Geometry check sheet. Reference: the model listing, model coordinates, mm. Face numbers are marked on the shaded views. A direction names the side the tool comes from. Round coordinates to 2 decimals unless told otherwise and drop trailing zeros. Loops run counter-clockwise (first coordinate to the right, second up) from the corner with the lowest first, then second, coordinate; pieces in that order, holes last.
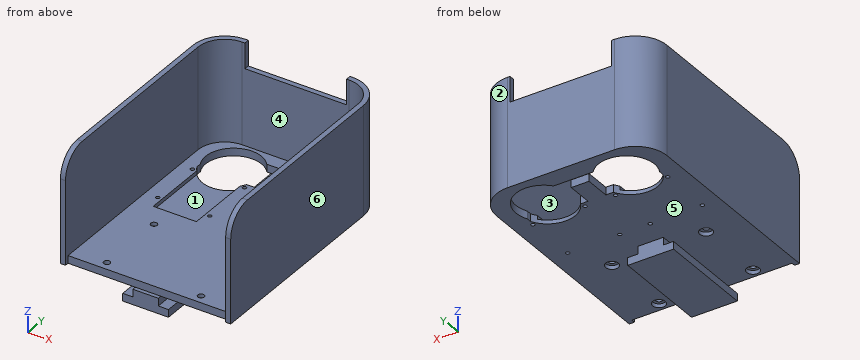
```python
from build123d import *

# Parameters (mm, degrees)
SKETCH_1_W           = 63
SKETCH_1_H           = 70
EXTRUDE_1_DEPTH      = 3
CUT_EXTRUDE_1_REACH  = 96.223
SKETCH_2_R           = 0.75
SKETCH_3_W           = 17
SKETCH_3_H           = 1.5
CUT_EXTRUDE_2_DEPTH  = 28
SKETCH_4_R           = 11
CUT_EXTRUDE_3_DEPTH  = 95.223139409
CUT_EXTRUDE_5_REACH  = 96.223
SKETCH_6_R           = 1.25
SKETCH_7_R           = 2.5
CUT_EXTRUDE_6_DEPTH  = 1.5
SKETCH_9_W           = 7
SKETCH_9_H           = 10
EXTRUDE_2_DEPTH      = 3
SKETCH_10_W          = 10
SKETCH_10_H          = 38
EXTRUDE_3_DEPTH      = 3
SKETCH_11_W          = 18
SKETCH_11_H          = 38
EXTRUDE_4_DEPTH      = 3
SKETCH_12_W          = 2
SKETCH_12_H          = 70
EXTRUDE_5_DEPTH      = 43
SWEEP_1_DEPTH        = 43
SWEEP_1_2_DEPTH      = 3
CUT_EXTRUDE_7_DEPTH  = 122.249642508
SKETCH_16_R          = 11
CUT_EXTRUDE_9_DEPTH  = 120.11538863
SKETCH_21_W          = 63
SKETCH_21_H          = 1.5
CUT_EXTRUDE_10_DEPTH = 3
CUT_EXTRUDE_11_REACH = 122.156
SKETCH_23_W          = 40
SKETCH_23_H          = 10


# Read off the part's stored shape, not the designer's step: the sweep step
with BuildPart() as part:
    # Sketch 1 → Extrude 1 (new body)
    with BuildSketch(Plane.XY):
        with Locations((31.5, 35)):
            Rectangle(SKETCH_1_W, SKETCH_1_H)
    extrude(amount=EXTRUDE_1_DEPTH)

    # Sketch 2 → Cut-Extrude 1 (cut, up to next)
    with BuildSketch(Plane.XY.offset(3), mode=Mode.PRIVATE) as cut_extrude_1_sk1:
        with Locations((5, 68)):
            Circle(SKETCH_2_R)
    cut_extrude_1_tool1 = extrude(cut_extrude_1_sk1.sketch, amount=-CUT_EXTRUDE_1_REACH, mode=Mode.PRIVATE) & part.part
    # Sketch 2 → Cut-Extrude 1 (cut, up to next)
    with BuildSketch(Plane.XY.offset(3), mode=Mode.PRIVATE) as cut_extrude_1_sk2:
        with Locations((5, 47.3)):
            Circle(SKETCH_2_R)
    cut_extrude_1_tool2 = extrude(cut_extrude_1_sk2.sketch, amount=-CUT_EXTRUDE_1_REACH, mode=Mode.PRIVATE) & part.part
    # Sketch 2 → Cut-Extrude 1 (cut, up to next)
    with BuildSketch(Plane.XY.offset(3), mode=Mode.PRIVATE) as cut_extrude_1_sk3:
        with Locations((25.5, 47.3)):
            Circle(SKETCH_2_R)
    cut_extrude_1_tool3 = extrude(cut_extrude_1_sk3.sketch, amount=-CUT_EXTRUDE_1_REACH, mode=Mode.PRIVATE) & part.part
    # Sketch 2 → Cut-Extrude 1 (cut, up to next)
    with BuildSketch(Plane.XY.offset(3), mode=Mode.PRIVATE) as cut_extrude_1_sk4:
        with Locations((25.5, 68)):
            Circle(SKETCH_2_R)
    cut_extrude_1_tool4 = extrude(cut_extrude_1_sk4.sketch, amount=-CUT_EXTRUDE_1_REACH, mode=Mode.PRIVATE) & part.part
    cut_extrude_1_1 = cut_extrude_1_tool1.solids().sort_by_distance((5, 68, 3))[0]
    add(cut_extrude_1_1, mode=Mode.SUBTRACT)
    cut_extrude_1_2 = cut_extrude_1_tool2.solids().sort_by_distance((5, 47.3, 3))[0]
    add(cut_extrude_1_2, mode=Mode.SUBTRACT)
    cut_extrude_1_3 = cut_extrude_1_tool3.solids().sort_by_distance((25.5, 47.3, 3))[0]
    add(cut_extrude_1_3, mode=Mode.SUBTRACT)
    cut_extrude_1_4 = cut_extrude_1_tool4.solids().sort_by_distance((25.5, 68, 3))[0]
    add(cut_extrude_1_4, mode=Mode.SUBTRACT)
    cut_extrude_1 = cut_extrude_1_1 + cut_extrude_1_2 + cut_extrude_1_3 + cut_extrude_1_4  # Cut-Extrude 1 as one shape, for the pattern or mirror that repeats it

    # Sketch 3 → Cut-Extrude 2 (cut)
    with BuildSketch(Plane(origin=(0, 70, 0), x_dir=(1, 0, 0), z_dir=(0, 1, 0))):
        with Locations((15.25, -2.25)):
            Rectangle(SKETCH_3_W, SKETCH_3_H)
    cut_extrude_2 = extrude(amount=-CUT_EXTRUDE_2_DEPTH, mode=Mode.SUBTRACT)

    # Sketch 4 → Cut-Extrude 3 (cut, through all)
    with BuildSketch(Plane(origin=(0, 0, 0), x_dir=(-1, 0, 0), z_dir=(0, 0, -1))):
        with Locations((-15.25, 75)):
            Circle(SKETCH_4_R)
    cut_extrude_3 = extrude(amount=-CUT_EXTRUDE_3_DEPTH, mode=Mode.SUBTRACT)

    # Mirror 1: Cut-Extrude 1, Cut-Extrude 2, Cut-Extrude 3 across plane
    add(cut_extrude_1.mirror(Plane.ZY.offset(-31.5)), mode=Mode.SUBTRACT)
    add(cut_extrude_2.mirror(Plane.ZY.offset(-31.5)), mode=Mode.SUBTRACT)
    add(cut_extrude_3.mirror(Plane.ZY.offset(-31.5)), mode=Mode.SUBTRACT)

    # Sketch 6 → Cut-Extrude 5 (cut, up to next)
    with BuildSketch(Plane(origin=(0, 0, 0), x_dir=(-1, 0, 0), z_dir=(0, 0, -1)), mode=Mode.PRIVATE) as cut_extrude_5_sk1:
        with Locations((-50, 5)):
            Circle(SKETCH_6_R)
    cut_extrude_5_tool1 = extrude(cut_extrude_5_sk1.sketch, amount=-CUT_EXTRUDE_5_REACH, mode=Mode.PRIVATE) & part.part
    # Sketch 6 → Cut-Extrude 5 (cut, up to next)
    with BuildSketch(Plane(origin=(0, 0, 0), x_dir=(-1, 0, 0), z_dir=(0, 0, -1)), mode=Mode.PRIVATE) as cut_extrude_5_sk2:
        with Locations((-50, 33)):
            Circle(SKETCH_6_R)
    cut_extrude_5_tool2 = extrude(cut_extrude_5_sk2.sketch, amount=-CUT_EXTRUDE_5_REACH, mode=Mode.PRIVATE) & part.part
    # Sketch 6 → Cut-Extrude 5 (cut, up to next)
    with BuildSketch(Plane(origin=(0, 0, 0), x_dir=(-1, 0, 0), z_dir=(0, 0, -1)), mode=Mode.PRIVATE) as cut_extrude_5_sk3:
        with Locations((-13, 33)):
            Circle(SKETCH_6_R)
    cut_extrude_5_tool3 = extrude(cut_extrude_5_sk3.sketch, amount=-CUT_EXTRUDE_5_REACH, mode=Mode.PRIVATE) & part.part
    # Sketch 6 → Cut-Extrude 5 (cut, up to next)
    with BuildSketch(Plane(origin=(0, 0, 0), x_dir=(-1, 0, 0), z_dir=(0, 0, -1)), mode=Mode.PRIVATE) as cut_extrude_5_sk4:
        with Locations((-13, 5)):
            Circle(SKETCH_6_R)
    cut_extrude_5_tool4 = extrude(cut_extrude_5_sk4.sketch, amount=-CUT_EXTRUDE_5_REACH, mode=Mode.PRIVATE) & part.part
    add(cut_extrude_5_tool1.solids().sort_by_distance((50, 5, 0))[0], mode=Mode.SUBTRACT)
    add(cut_extrude_5_tool2.solids().sort_by_distance((50, 33, 0))[0], mode=Mode.SUBTRACT)
    add(cut_extrude_5_tool3.solids().sort_by_distance((13, 33, 0))[0], mode=Mode.SUBTRACT)
    add(cut_extrude_5_tool4.solids().sort_by_distance((13, 5, 0))[0], mode=Mode.SUBTRACT)

    # Sketch 7 → Cut-Extrude 6 (cut)
    with BuildSketch(Plane(origin=(0, 0, 0), x_dir=(-1, 0, 0), z_dir=(0, 0, -1))):
        with Locations((-50, 33)):
            Circle(SKETCH_7_R)
        with Locations((-13, 33)):
            Circle(SKETCH_7_R)
        with Locations((-13, 5)):
            Circle(SKETCH_7_R)
        with Locations((-50, 5)):
            Circle(SKETCH_7_R)
    extrude(amount=-CUT_EXTRUDE_6_DEPTH, mode=Mode.SUBTRACT)

    # Sketch 9 → Extrude 2 (add)
    with BuildSketch(Plane(origin=(0, 0, 0), x_dir=(-1, 0, 0), z_dir=(0, 0, -1))):
        with Locations((-31.5, 75)):
            Rectangle(SKETCH_9_W, SKETCH_9_H)
    extrude(amount=-EXTRUDE_2_DEPTH)

    # Sketch 10 → Extrude 3 (add)
    with BuildSketch(Plane(origin=(0, 0, 0), x_dir=(-1, 0, 0), z_dir=(0, 0, -1))):
        with Locations((-31.5, 19)):
            Rectangle(SKETCH_10_W, SKETCH_10_H)
    extrude(amount=EXTRUDE_3_DEPTH)

    # Sketch 11 → Extrude 4 (add)
    with BuildSketch(Plane(origin=(0, 0, -3), x_dir=(-1, 0, 0), z_dir=(0, 0, -1))):
        with Locations((-31.5, 19)):
            Rectangle(SKETCH_11_W, SKETCH_11_H)
    extrude(amount=EXTRUDE_4_DEPTH)

    # Sketch 12 → Extrude 5 (add)
    with BuildSketch(Plane(origin=(0, 0, 0), x_dir=(-1, 0, 0), z_dir=(0, 0, -1))):
        with Locations((-64, 35)):
            Rectangle(SKETCH_12_W, SKETCH_12_H)
        with Locations((1, 35)):
            Rectangle(SKETCH_12_W, SKETCH_12_H)
    extrude(amount=-EXTRUDE_5_DEPTH)

    # Sweep 1 outline → Sweep 1 (add)
    with BuildSketch(Plane.XY):
        with BuildLine():
            ThreePointArc((52.547958971, 89.452041029), (59.93866806, 86.390709089), (63, 79))
            Line((63, 79), (63, 70))
            Line((63, 70), (65, 70))
            Line((65, 70), (65, 79))
            ThreePointArc((65, 79), (61.352881622, 87.804922651), (52.547958971, 91.452041029))
            Line((52.547958971, 91.452041029), (10.452041029, 91.452041029))
            ThreePointArc((10.452041029, 91.452041029), (1.647118378, 87.804922651), (-2, 79))
            Line((-2, 79), (-2, 70))
            Line((-2, 70), (0, 70))
            Line((0, 70), (0, 79))
            ThreePointArc((0, 79), (3.06133194, 86.390709089), (10.452041029, 89.452041029))
            Line((10.452041029, 89.452041029), (52.547958971, 89.452041029))
        make_face()
    extrude(amount=SWEEP_1_DEPTH)

    # Sweep 1 2 outline → Sweep 1 2 (add)
    with BuildSketch(Plane.XY):
        with BuildLine():
            Line((63, 70), (63, 79))
            ThreePointArc((63, 79), (59.93866806, 86.390709089), (52.547958971, 89.452041029))
            Line((52.547958971, 89.452041029), (10.452041029, 89.452041029))
            ThreePointArc((10.452041029, 89.452041029), (3.06133194, 86.390709089), (0, 79))
            Line((0, 79), (0, 70))
            Line((0, 70), (5.452041029, 70))
            Line((5.452041029, 70), (5.452041029, 79))
            ThreePointArc((5.452041029, 79), (6.916507123, 82.535533906), (10.452041029, 84))
            Line((10.452041029, 84), (52.547958971, 84))
            ThreePointArc((52.547958971, 84), (56.083492877, 82.535533906), (57.547958971, 79))
            Line((57.547958971, 79), (57.547958971, 70))
            Line((57.547958971, 70), (63, 70))
        make_face()
    extrude(amount=SWEEP_1_2_DEPTH)

    # Sketch 15 → Cut-Extrude 7 (cut, through all)
    with BuildSketch(Plane.ZY.offset(2)):
        with BuildLine():
            ThreePointArc((43, 10), (40.071067812, 2.928932188), (33, 0))
            Line((33, 0), (43, 0))
            Line((43, 0), (43, 10))
        make_face()
    extrude(amount=-CUT_EXTRUDE_7_DEPTH, mode=Mode.SUBTRACT)

    # Sketch 16 → Cut-Extrude 9 (cut, through all)
    with BuildSketch(Plane.XY.offset(3)):
        with Locations((15.25, 77)):
            Circle(SKETCH_16_R)
        with Locations((47.75, 77)):
            Circle(SKETCH_16_R)
    extrude(amount=-CUT_EXTRUDE_9_DEPTH, mode=Mode.SUBTRACT)

    # Sketch 21 → Cut-Extrude 10 (cut)
    with BuildSketch(Plane.XY.offset(3)):
        with Locations((31.5, 0.75)):
            Rectangle(SKETCH_21_W, SKETCH_21_H)
    extrude(amount=-CUT_EXTRUDE_10_DEPTH, mode=Mode.SUBTRACT)

    # Sketch 23 → Cut-Extrude 11 (cut, up to next)
    with BuildSketch(Plane(origin=(0, 91.452041029, 0), x_dir=(1, 0, 0), z_dir=(0, 1, 0)), mode=Mode.PRIVATE) as cut_extrude_11_sk1:
        with Locations((31.5, -38)):
            Rectangle(SKETCH_23_W, SKETCH_23_H)
    cut_extrude_11_tool1 = extrude(cut_extrude_11_sk1.sketch, amount=-CUT_EXTRUDE_11_REACH, mode=Mode.PRIVATE) & part.part
    add(cut_extrude_11_tool1.solids().sort_by_distance((31.5, 91.452041, 38))[0], mode=Mode.SUBTRACT)


solid = part.part
```
1) Mould release check, pull along X, two halves, no side actions. Record for the marked faces 4, 5 and 6: +X half, -X half, draft (parallel to the pull), parting line (faces both ways), or undercut.
Report:
face 4: undercut
face 5: draft
face 6: +X half
2) Sectioned sample at A-A, the plane y = 33. State how many separate pieces and enclosed holes the cut face has, then the cut area to 4 significant figures.
Report:
separate pieces: 3
enclosed holes: 0
area: 422.5 mm2
3) Scan lines: line 1 along X through (y, z) = (19, 12); line 2 along Y through (x, z) = (37, 2); line 3 along Y through (x, z) = (37.5, 1.65). Record each from-to range of solid material in increasing order.
Report:
line 1: x = -2 to 0, 63 to 65
line 2: y = 1.5 to 46.74, 47.86 to 67.44, 68.56 to 70, 84 to 91.45
line 3: y = 1.5 to 46.55, 48.05 to 67.25, 68.75 to 70, 84 to 91.45
4) Access from +Z, -Z, +X, -X, +Y, -Y to the whole of each face (thin tool, end or side, straight path). Record for the marked faces 1, 2 and 3.
Report:
face 1: +Z
face 2: +Z, -Z, +X, +Y
face 3: +Z, -Y
5) Sectioned sample at C-C, the plane x = 50. Record the cut outline in (y, z), then the cut area to 3 significant figures.
Report:
outline: (1.5, 0) - (2.5, 0) - (2.5, 1.5) - (3.75, 1.5) - (3.75, 3) - (1.5, 3) - close; (6.25, 1.5) - (7.5, 1.5) - (7.5, 0) - (30.5, 0) - (30.5, 1.5) - (31.75, 1.5) - (31.75, 3) - (6.25, 3) - close; (34.25, 1.5) - (35.5, 1.5) - (35.5, 0) - (64.23, 0) - (64.23, 1.5) - (42, 1.5) - (42, 3) - (34.25, 3) - close; (87.77, 0) - (91.45, 0) - (91.45, 33) - (89.45, 33) - (89.45, 3) - (87.77, 3) - close
area: 203 mm2
6) Sectioned sample at D-D, the plane y = 81. Record the cut outline in (x, z).
Report:
outline: (-1.84, 0) - (5, 0) - (5, 3) - (0.19, 3) - (0.19, 43) - (-1.84, 43) - close; (58, 0) - (64.84, 0) - (64.84, 43) - (62.81, 43) - (62.81, 3) - (58, 3) - close
7) Sectioned sample at B-B, the plane z = 30.5. Record the cut outline in (x, y), then the cut area to 3 significant figures.
Report:
outline: (-2, 0) - (0, 0) - (0, 79) arc R10.45 cw to (10.45, 89.45) - (52.55, 89.45) arc R10.45 cw to (63, 79) - (63, 0) - (65, 0) - (65, 79) arc R12.45 ccw to (52.55, 91.45) - (10.45, 91.45) arc R12.45 ccw to (-2, 79) - close
area: 472 mm2
8) Gauge pin test, flat ends, axial feed: pin 1 (8.5 mm diameter, centred on x = 44, y = 60, fed in from +Z); pin 2 (4 mm diameter, centred on x = 32, y = 29.5, fed in from +Z); pin 3 (2 mm diameter, centred on x = 47.5, z = 32.5, fed in from -Y); pin 4 (1.2 mm diameter, centred on x = 37.5, y = 47.3, fed in from +Z). Record the tip position at first contact, or that the pin passes through.
Report:
pin 1: stops at z = 1.5
pin 2: stops at z = 3
pin 3: stops at y = 89.45
pin 4: passes through
